```python
from build123d import *

# Parameters (mm, degrees)
SKETCH1_R           = 1.25
SKETCH1_W           = 25
SKETCH1_H           = 25
BOSS_EXTRUDE1_DEPTH = 3
SKETCH2_R           = 0.5
CUT_EXTRUDE1_DEPTH  = 10


with BuildPart() as part:
    # Sketch1 → Boss-Extrude1 (new body)
    with BuildSketch(Plane.XY):
        with BuildLine():
            Line((-33.221634358, 0.474846268), (-24.289446699, 2.749498978))
            ThreePointArc((-24.289446699, 2.749498978), (-18.546247277, 12.304618098), (-9.045759802, 18.137745796))
            Line((-9.045759802, 18.137745796), (-6.684093846, 27.047322398))
            ThreePointArc((-6.684093846, 27.047322398), (-1.851003919, 30.766212818), (2.982086008, 27.047322398))
            Line((2.982086008, 27.047322398), (5.343751964, 18.137745796))
            ThreePointArc((5.343751964, 18.137745796), (14.844239439, 12.304618098), (20.587438861, 2.749498978))
            Line((20.587438861, 2.749498978), (29.51962652, 0.474846268))
            ThreePointArc((29.51962652, 0.474846268), (33.2856667, -4.393192656), (29.475612525, -9.226860909))
            Line((29.475612525, -9.226860909), (20.523154011, -11.420375867))
            ThreePointArc((20.523154011, -11.420375867), (14.686585816, -20.929838384), (5.121898214, -26.675459041))
            Line((5.121898214, -26.675459041), (3.016856108, -35.649132707))
            ThreePointArc((3.016856108, -35.649132707), (-1.851003919, -39.507231329), (-6.718863946, -35.649132707))
            Line((-6.718863946, -35.649132707), (-8.823906053, -26.675459041))
            ThreePointArc((-8.823906053, -26.675459041), (-18.388593654, -20.929838384), (-24.225161849, -11.420375867))
            Line((-24.225161849, -11.420375867), (-33.177620364, -9.226860909))
            ThreePointArc((-33.177620364, -9.226860909), (-36.987674539, -4.393192656), (-33.221634358, 0.474846268))
        make_face()
        with Locations((-1.851003919, 25.766212818)):
            Circle(SKETCH1_R, mode=Mode.SUBTRACT)
        with Locations((28.148996081, -4.233787182)):
            Circle(SKETCH1_R, mode=Mode.SUBTRACT)
        with Locations((-1.851003919, -34.233787182)):
            Circle(SKETCH1_R, mode=Mode.SUBTRACT)
        with Locations((-31.851003919, -4.233787182)):
            Circle(SKETCH1_R, mode=Mode.SUBTRACT)
        with Locations((-3.613074624, -2.60843855)):
            Rectangle(SKETCH1_W, SKETCH1_H, mode=Mode.SUBTRACT)
    extrude(amount=BOSS_EXTRUDE1_DEPTH)

    # Sketch2 → Cut-Extrude1 (cut)
    with BuildSketch(Plane.XY.offset(3)):
        with Locations((-16.113074624, 9.89156145)):
            Circle(SKETCH2_R)
        with Locations((8.886925376, 9.89156145)):
            Circle(SKETCH2_R)
        with Locations((8.886925376, -15.10843855)):
            Circle(SKETCH2_R)
        with Locations((-16.113074624, -15.10843855)):
            Circle(SKETCH2_R)
    extrude(amount=-CUT_EXTRUDE1_DEPTH, mode=Mode.SUBTRACT)


solid = part.part
```
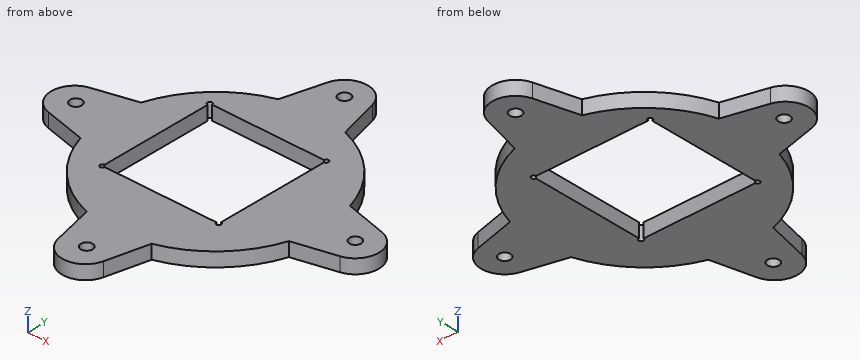
Model file for the job. Use its own axes, mm. Coordinates: 2 decimals unless noted, no trailing zeros. Loops run counter-clockwise (first coordinate to the right, second up) from the corner with the lowest first, then second, coordinate; pieces in that order, holes last. Notation, with made-up numbers: (8, 46.5) - (13, 46.5) arc R22 cw to (13, 73.5) - close; hole circle Ø4 at (22.5, 49). An arc over 180 degrees is marked (long way). Answer as a JSON object with one key per item and string values. Group by question number.
(1) Cut at D-D (x = -27). Give the cut face in (y, z), then the cut area to 3 significant figures.
(2) Probe line 1 along Y through (x, z) = (-5, 2.2); line 2 along Y through (x, z) = (7.5, 2.2); line 3 along X through (y, z) = (-2.5, 1.3). List the from-to ranges inside material, lowest first.
(3) Flat gauge pin, fed straight in: pin 1 (1 mm diameter, centred on x = 1, z = 1.5, fed in from +Y). Where does the tip first touch, or does it go through?
(4) Cut at A-A (x = 0.5). Give the cut face in (y, z), then the cut area to 3 significant figures.
(5) Cut at C-C (z = 1.35). Give the cut face in (x, y), then the cut area to 3 significant figures.
(6) Cut at B-B (y = -13). Give the cut face in (x, z).
Geometry says:
{
 "1": {"outline": "(-10.74, 0) - (2.06, 0) - (2.06, 3) - (-10.74, 3) - close", "area": "38.4 mm^2"},
 "2": {"line 1": "y = -38.39 to -15.11, 9.89 to 29.65", "line 2": "y = -25.79 to -15.11, 9.89 to 17.33", "line 3": "x = -36.62 to -16.11, 8.89 to 32.92"},
 "3": {"pin 1": "stops at y = 30.18"},
 "4": {"outline": "(-38.92, 0) - (-15.11, 0) - (-15.11, 3) - (-38.92, 3) - close; (9.89, 0) - (30.18, 0) - (30.18, 3) - (9.89, 3) - close", "area": "132 mm^2"},
 "5": {"outline": "(-33.22, 0.47) arc R5 ccw to (-33.18, -9.23) - (-24.23, -11.42) arc R23.5 ccw to (-8.82, -26.68) - (-6.72, -35.65) arc R5 ccw to (3.02, -35.65) - (5.12, -26.68) arc R23.5 ccw to (20.52, -11.42) - (29.48, -9.23) arc R5 ccw to (29.52, 0.47) - (20.59, 2.75) arc R23.5 ccw to (5.34, 18.14) - (2.98, 27.05) arc R5 ccw to (-6.68, 27.05) - (-9.05, 18.14) arc R23.5 ccw to (-24.29, 2.75) - close; hole circle Ø2.5 at (-31.85, -4.23); hole (-16.11, -14.61) arc R0.5 ccw (long way) to (-15.61, -15.11) - (8.39, -15.11) arc R0.5 ccw (long way) to (8.89, -14.61) - (8.89, 9.39) arc R0.5 ccw (long way) to (8.39, 9.89) - (-15.61, 9.89) arc R0.5 ccw (long way) to (-16.11, 9.39) - close; hole circle Ø2.5 at (-1.85, -34.23); hole circle Ø2.5 at (-1.85, 25.77); hole circle Ø2.5 at (28.15, -4.23)", "area": "1,580 mm^2"},
 "6": {"outline": "(-23.65, 0) - (-16.11, 0) - (-16.11, 3) - (-23.65, 3) - close; (8.89, 0) - (19.95, 0) - (19.95, 3) - (8.89, 3) - close"}
}
